from build123d import *

# Parameters (mm, degrees)
SKETCH1_R           = 9
SKETCH1_R_2         = 7.5
SKETCH1_R_3         = 4
BOSS_EXTRUDE1_DEPTH = 2
SKETCH1_3_R         = 9
SKETCH1_3_R_2       = 7.5
BOSS_EXTRUDE2_DEPTH = 7
BOSS_EXTRUDE3_DEPTH = 27
FILLET1_R           = 2


with BuildPart() as part:
    # Sketch1 → Boss-Extrude1 (new body)
    # profile 1 of 6: a face of its own
    with BuildSketch(Plane.XY):
        with BuildLine():
            ThreePointArc((28.428715875, 22.086378465), (32.999839448, 18.790712656), (38.627105052, 18.489937528))
            ThreePointArc((38.627105052, 18.489937528), (62, 0), (38.627105052, -18.489937528))
            ThreePointArc((38.627105052, -18.489937528), (32.999839448, -18.790712656), (28.428715875, -22.086378465))
            ThreePointArc((28.428715875, -22.086378465), (-36, 0), (28.428715875, 22.086378465))
        make_face()
        with BuildLine():
            ThreePointArc((26.059656218, 20.245846927), (-33, 0), (26.059656218, -20.245846927))
            ThreePointArc((26.059656218, -20.245846927), (32.002116864, -15.961481374), (39.317562149, -15.570473707))
            ThreePointArc((39.317562149, -15.570473707), (59, 0), (39.317562149, 15.570473707))
            ThreePointArc((39.317562149, 15.570473707), (32.002116864, 15.961481374), (26.059656218, 20.245846927))
        make_face(mode=Mode.SUBTRACT)
    # profile 2 of 6: a face of its own
    with BuildSketch(Plane.XY):
        with BuildLine():
            ThreePointArc((26.059656218, 20.245846927), (32.002116864, 15.961481374), (39.317562149, 15.570473707))
            ThreePointArc((39.317562149, 15.570473707), (59, 0), (39.317562149, -15.570473707))
            ThreePointArc((39.317562149, -15.570473707), (32.002116864, -15.961481374), (26.059656218, -20.245846927))
            ThreePointArc((26.059656218, -20.245846927), (-33, 0), (26.059656218, 20.245846927))
        make_face()
        with Locations((43, 0)):
            Circle(SKETCH1_R, mode=Mode.SUBTRACT)
        Circle(SKETCH1_R, mode=Mode.SUBTRACT)
    # profile 3 of 6: a face of its own
    with BuildSketch(Plane.XY):
        Circle(SKETCH1_R)
        Circle(SKETCH1_R_2, mode=Mode.SUBTRACT)
    # profile 4 of 6: a face of its own
    with BuildSketch(Plane.XY):
        Circle(SKETCH1_R_2)
        Circle(SKETCH1_R_3, mode=Mode.SUBTRACT)
    # profile 5 of 6: a face of its own
    with BuildSketch(Plane.XY):
        with Locations((43, 0)):
            Circle(SKETCH1_R)
        with Locations((43, 0)):
            Circle(SKETCH1_R_2, mode=Mode.SUBTRACT)
    # profile 6 of 6: a face of its own
    with BuildSketch(Plane.XY):
        with Locations((43, 0)):
            Circle(SKETCH1_R_2)
        with Locations((43, 0)):
            Circle(SKETCH1_R_3, mode=Mode.SUBTRACT)
    extrude(amount=BOSS_EXTRUDE1_DEPTH)

    # Sketch1_3 → Boss-Extrude2 (add)
    # profile 1 of 2: a face of its own
    with BuildSketch(Plane.XY):
        Circle(SKETCH1_3_R)
        Circle(SKETCH1_3_R_2, mode=Mode.SUBTRACT)
    # profile 2 of 2: a face of its own
    with BuildSketch(Plane.XY):
        with Locations((43, 0)):
            Circle(SKETCH1_3_R)
        with Locations((43, 0)):
            Circle(SKETCH1_3_R_2, mode=Mode.SUBTRACT)
    extrude(amount=BOSS_EXTRUDE2_DEPTH)

    # Sketch1_4 → Boss-Extrude3 (add)
    with BuildSketch(Plane.XY):
        with BuildLine():
            ThreePointArc((28.428715875, 22.086378465), (32.999839448, 18.790712656), (38.627105052, 18.489937528))
            ThreePointArc((38.627105052, 18.489937528), (62, 0), (38.627105052, -18.489937528))
            ThreePointArc((38.627105052, -18.489937528), (32.999839448, -18.790712656), (28.428715875, -22.086378465))
            ThreePointArc((28.428715875, -22.086378465), (-36, 0), (28.428715875, 22.086378465))
        make_face()
        with BuildLine():
            ThreePointArc((26.059656218, 20.245846927), (-33, 0), (26.059656218, -20.245846927))
            ThreePointArc((26.059656218, -20.245846927), (32.002116864, -15.961481374), (39.317562149, -15.570473707))
            ThreePointArc((39.317562149, -15.570473707), (59, 0), (39.317562149, 15.570473707))
            ThreePointArc((39.317562149, 15.570473707), (32.002116864, 15.961481374), (26.059656218, 20.245846927))
        make_face(mode=Mode.SUBTRACT)
    extrude(amount=BOSS_EXTRUDE3_DEPTH)

    # Fillet1
    fillet1_edges = [part.edges().sort_by_distance(p)[0] for p in [
        (-36, 0, 0),
        (32.999839448, 18.790712656, 0),
        (32.002116864, 15.961481374, 2),
        (-33, 0, 2),
        (59, 0, 2),
        (32.002116864, -15.961481374, 2),
        (62, 0, 0),
        (32.999839448, -18.790712656, 0),
    ]]
    fillet(fillet1_edges, radius=FILLET1_R)


solid = part.part
Work out the finished part from the listing and answer in its coordinate system (mm). A direction names the side the tool comes from. Give positions to 0.01 mm unless a question says otherwise; leave off trailing zeros. Loops run counter-clockwise (first coordinate to the right, second up) from the corner with the lowest first, then second, coordinate; pieces in that order, holes last. Notation, with made-up numbers: (57, -16.5) - (79, -16.5) arc R21 ccw to (79, -8.5) - close; hole circle Ø9 at (-38.75, -33). An arc over 180 degrees is marked (long way). Answer in a Markdown table with one row per item.
(1) Flat-ended cylindrical pins translate along their axes: pin 1 Ø12 at (x, z) = (15, 23.5) entering from +Y; pin 2 Ø9 at (x, y) = (-3.5, 1) entering from +Z; pin 3 Ø4.5 at (x, y) = (-2.5, 3.5) entering from +Z; pin 4 Ø7 at (x, y) = (0, 0) entering from -Z. Find the tip coordinate at first contact, or state that the pin passes through.
Results list:
| item | result |
|---|---|
| pin 1 | stops at y = 34.86 |
| pin 2 | stops at z = 7 |
| pin 3 | stops at z = 2 |
| pin 4 | passes through |
(2) Section C-C (z = 8.75) is taken. Give the vertices of the cut face in (x, y).
Results list:
| item | result |
|---|---|
| outline | (28.43, -22.09) arc R10 cw to (38.63, -18.49) arc R19 ccw (long way) to (38.63, 18.49) arc R10 cw to (28.43, 22.09) arc R36 ccw (long way) to start; hole (26.06, -20.25) arc R13 cw to (39.32, -15.57) arc R16 ccw (long way) to (39.32, 15.57) arc R13 cw to (26.06, 20.25) arc R33 ccw (long way) to start |
(3) Section B-B (y = 0) is taken. State how many separate pieces and enclosed holes the cut face has, and give its area (3 significant figures).
Results list:
| item | result |
|---|---|
| separate pieces | 3 |
| enclosed holes | 0 |
| area | 344 mm² |
(4) Consider L1, parallel to Y at x = 43, z = 5.75; L2, parallel to Y at x = 43, z = 16.75; L3, parallel to Y at x = 0, z = 16.5. Determine where each line is inside the solid, lowest interval first. Write a range as [from, to].
Results list:
| item | result |
|---|---|
| L1 | y = [-19, -16], [-9, -7.5], [7.5, 9], [16, 19] |
| L2 | y = [-19, -16], [16, 19] |
| L3 | y = [-36, -33], [33, 36] |
(5) Section A-A (z = 3) is taken. Give the vertices of the cut face in (x, y).
Results list:
| item | result |
|---|---|
| outline | circle Ø18 at (0, 0); (28.43, -22.09) arc R10 cw to (38.63, -18.49) arc R19 ccw (long way) to (38.63, 18.49) arc R10 cw to (28.43, 22.09) arc R36 ccw (long way) to start; circle Ø18 at (43, 0); hole circle Ø15 at (0, 0); hole (25.85, -20.08) arc R13.27 cw to (39.38, -15.31) arc R15.73 ccw (long way) to (39.38, 15.31) arc R13.27 cw to (25.85, 20.08) arc R32.73 ccw (long way) to start; hole circle Ø15 at (43, 0) |
(6) For a pull along Y with two mould halves and no side action, classify faces 1 (the face through (-35.98, -1.25, 14.32)), 2 (the face through (-2, 7.4, 7)), 3 (the face through (32.92, 18.82, 14.32)) as pulls with the +Y half, pulls with the -Y half, needs draft (parallel to the pull), parting line crosses it, or undercut.
Results list:
| item | result |
|---|---|
| face 1 | parting line crosses it |
| face 2 | undercut |
| face 3 | pulls with the +Y half |
(7) A tool of negligible diameter and unlimited length cuts with its end or side. For faces 4 (the face through (62, 0, 14)), 5 (the face through (-1.172, 8.923, 4.465)), from which of +Z, -Z, +X, -X, +Y, -Y can it reach the whole face along a straight path? Write none if from no direction.
Results list:
| item | result |
|---|---|
| face 4 | +Z, -Z |
| face 5 | +Z |
